Input: part model. Units: mm. Frame: model coordinates. Face numbers are marked on the shaded views. A direction names the side the tool comes from. Give positions to 0.01 mm unless a question says otherwise; leave off trailing zeros. Write each loop counter-clockwise with the first axis right and the second up, starting at its lowest first coordinate (ties: lowest second). Pieces come first, ordered by that corner, then holes.
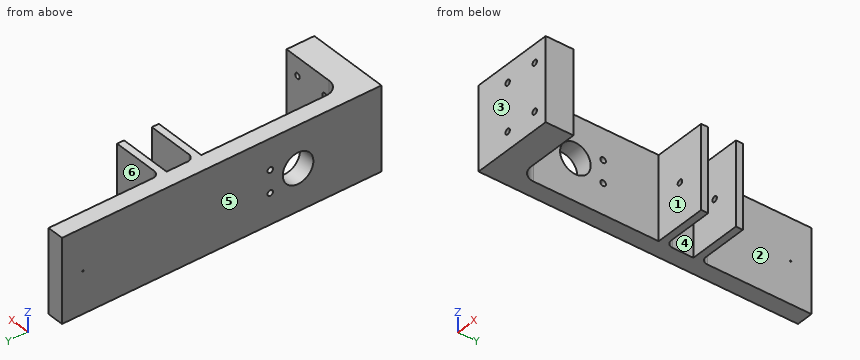
Autodesk Inventor part; units mm, degrees
ref_plane "YZ Plane" through (0, 0, 0) normal (1, 0, 0) x (0, 1, 0)
ref_plane "XZ Plane" through (0, 0, 0) normal (0, 1, 0) x (-1, 0, 0)
ref_plane "XY Plane" through (0, 0, 0) normal (0, 0, 1) x (1, 0, 0)
sketch "Эскиз1" plane through (0, 0, 0) normal (0, 1, 0) x (-1, 0, 0)
  line L0 (0, 0) -> (-60, 0)
  line L1 (-60, 0) -> (-60, -60)
  line L2 (-60, -60) -> (0, -60)
  line L3 (0, -60) -> (0, 0)
  dimension "d0" = 60
  dimension "d1" = 60
extrude "Выдавливание1" add sketch "Эскиз1" along normal blind 20
sketch "Эскиз2" plane through (0, 20, 0) normal (0, 1, 0) x (1, 0, 0)
  line L0 (0, 0) -> (60, 0)
  line L1 (0, 0) -> (12, 0)
  line L2 (12, 0) -> (12, 60)
  line L3 (60, 60) -> (0, 60)
  line L4 (0, 60) -> (0, 0)
  line L5 (0, 60) -> (0, 0)
  dimension "d4" = 12
extrude "Выдавливание2" add sketch "Эскиз2" along normal blind 260
sketch "Эскиз3" plane through (0, 20, 0) normal (0, 1, 0) x (1, 0, 0)
  point P0 (0, 0)
  point P1 (26, 13)
  point P2 (26, 47)
  point P3 (50.2241, 13)
  point P4 (50.2241, 47)
hole "Отверстие1" at (26, 20, -13) at (26, 20, -47) at (50.2241, 20, -13) at (50.2241, 20, -47) direction (0, -1, 0) diameter 4 depth 40 tip angle 118
sketch "Эскиз4" plane through (12, 20, 0) normal (1, 0, 0) x (0, 0, -1)
  point P0 (0, -20)
  point P1 (30, 88)
  dimension "d14" = 0
extrude "Выдавливание3" [suppressed]
sketch "Эскиз5" plane through (12, 20, 0) normal (1, 0, 0) x (0, 0, -1)
  point P0 (0, -20)
sketch "Эскиз6" plane through (0, 0, 0) normal (0, 0, 1) x (1, 0, 0)
  line L0 (0, 0) -> (0, 280)
  line L1 (12, 20) -> (12, 280)
sketch "Эскиз7" plane through (60, 0, -60) normal (0, 0, -1) x (-1, 0, 0)
  point P0 (60, 0)
sketch "Эскиз8" plane through (12, 20, 0) normal (1, 0, 0) x (0, 0, -1)
  circle A0 centre (30, 80) radius 11.5
  point P0 (0, -20)
  point P1 (0, 80)
  dimension "d17" = 23
extrude "Выдавливание4" cut sketch "Эскиз8" against normal blind 100
sketch "Эскиз9" plane through (0, 0, -60) normal (-1, 0, 0) x (0, 0, 1)
  circle A0 centre (29.731, 99.8395) radius 12.5286
  point P0 (60, 0)
  point P1 (0, 80)
extrude "Выдавливание5" add sketch "Эскиз9" against normal blind 12
sketch "Эскиз10" plane through (0, 0, -60) normal (-1, 0, 0) x (0, 0, 1)
  line L0 (0, 0) -> (0, 280)
  circle A0 centre (30, 60) radius 11
  circle A1 centre (22, 80) radius 2
  circle A2 centre (38, 80) radius 2
  point P0 (60, 0)
  point P1 (0, 60)
  point P2 (0, 80)
  point P3 (30, 80)
  dimension "d22" = 22
  dimension "d23" = 4
  dimension "d24" = 4
extrude "Выдавливание6" cut sketch "Эскиз10" against normal blind 12
sketch "Эскиз11" plane through (0, 0, 0) normal (0, -1, 0) x (1, 0, 0)
  point P0 (0, 0)
fillet "Сопряжение1" radius 10 1 edges at (12, 20, -30)
sketch "Эскиз12" plane through (0, 0, -60) normal (-1, 0, 0) x (0, 0, 1)
  line L0 (0, 120) -> (60, 120)
  line L1 (60, 120) -> (60, 125)
  line L2 (60, 125) -> (0, 125)
  line L3 (0, 125) -> (0, 120)
  point P0 (60, 0)
  dimension "d28" = 60
  dimension "d29" = 5
extrude "Выдавливание7" add sketch "Эскиз12" against normal blind 50
fillet "Сопряжение2" radius 5 1 edges at (12, 125, -30)
sketch "Эскиз13" plane through (50, 125, 0) normal (0, 1, 0) x (1, 0, 0)
  circle A0 centre (-19, 30) radius 2
  point P0 (-50, 0)
  dimension "d33" = 4
extrude "Выдавливание8" cut sketch "Эскиз13" against normal blind 50
sketch "Эскиз14" plane through (0, 0, -60) normal (-1, 0, 0) x (0, 0, 1)
  line L0 (0, 0) -> (0, 280)
  line L1 (0, 145) -> (60, 145)
  line L2 (60, 145) -> (60, 150)
  line L3 (60, 150) -> (0, 150)
  line L4 (0, 150) -> (0, 145)
  point P0 (60, 0)
  dimension "d36" = 60
  dimension "d37" = 5
extrude "Выдавливание9" add sketch "Эскиз14" against normal blind 50
fillet "Сопряжение3" radius 5 1 edges at (12, 150, -30)
sketch "Эскиз15" plane through (12, 145, -60) normal (0, -1, 0) x (1, 0, 0)
  circle A0 centre (19, 30) radius 2
  circle A1 centre (19, 30) radius 2
  circle A2 centre (19, 30) radius 2
  point P0 (-12, 60)
  point P1 (3.4297, 11.4015)
  dimension "d41" = 4
extrude "Выдавливание10" cut sketch "Эскиз15" against normal blind 50
sketch "Эскиз16" plane through (0, 0, -60) normal (-1, 0, 0) x (0, 0, 1)
  line L0 (0, 0) -> (0, 280)
  circle A0 centre (30, 215) radius 0.5
  point P0 (60, 0)
  point P1 (0, 215)
  point P2 (0, 215)
  dimension "d44" = 1
extrude "Выдавливание11" cut sketch "Эскиз16" against normal blind 100
sketch "Эскиз17" plane through (12, 280, 0) normal (1, 0, 0) x (0, 0, -1)
  point P0 (0, -280)
sketch "Эскиз18" plane through (12, 280, 0) normal (1, 0, 0) x (0, 0, -1)
  line L0 (0, -125) -> (0, 0)
  line L1 (60, -280) -> (60, 0)
  line L2 (0, -80) -> (0, -50)
  line L3 (0, -50) -> (5, -50)
  line L4 (5, -50) -> (5, -80)
  line L5 (5, -80) -> (0, -80)
  line L6 (0, -80) -> (0, -50)
  point P0 (0, -280)
  point P1 (30, -80)
  point P2 (30, -50)
  dimension "d47" = 5
extrude "Выдавливание12" add sketch "Эскиз18" along normal blind 44.5
sketch "Эскиз19" plane through (0, 0, 0) normal (0, 0, 1) x (1, 0, 0)
  circle A0 centre (52.5, 223) radius 2
  circle A1 centre (52.5, 207) radius 2
  point P0 (0, 0)
  point P1 (52.5, 215)
  dimension "d50" = 4
  dimension "d51" = 4
extrude "Выдавливание13" cut sketch "Эскиз19" against normal blind 45
fillet "Сопряжение4" radius 10 1 edges at (12, 215, -5)
sketch "Эскиз20" plane through (12, 280, 0) normal (1, 0, 0) x (0, 0, -1)
  line L0 (0, -280) -> (0, 0)
  line L1 (0, -50.033) -> (60, -50.033)
  line L2 (60, -280) -> (60, 0)
  line L3 (60, -50.033) -> (60, 0)
  line L4 (60, 0) -> (0, 0)
  line L5 (0, 0) -> (0, -50.033)
extrude "Выдавливание14" cut sketch "Эскиз20" against normal blind 100
sketch "Эскиз21" plane through (0, 0, 0) normal (0, 0, 1) x (1, 0, 0)
  line L0 (22, 230) -> (12, 230)
  line L1 (22, 200) -> (56.5, 200)
  line L2 (12, 230) -> (56.5, 230)
  line L3 (56.5, 230) -> (56.5, 200)
  line L4 (56.5, 200) -> (12, 200)
  line L5 (12, 200) -> (12, 230)
  point P0 (0, 0)
extrude "Выдавливание15" cut sketch "Эскиз21" against normal blind 100
properties part number "Подпора"
Q1. Section B-B, the plane y = 80. Return the cut outline in (x, z).
Q2. Section A-A, the plane x = 26. Return the cut outline in (y, z).
Q3. Mould query, pull axis Y, two halves, no side actions, for the marked faces 4, 5 and 6. Classes: +Y half, -Y half, draft (parallel to the pull), parting line (faces both ways), or undercut.
Q4. Pin query (flat end, axial travel): pin 1 (6.5 mm diameter, centred on x = 50.22, z = -47, fed in from +Y); pin 2 (16.5 mm diameter, centred on y = 138, z = -24, fed in from +X); pin 3 (6 mm diameter, centred on y = 168.5, z = -53, fed in from +X). Return the tip coordinate at first contact, or that it passes through.
Q5. Section C-C, the plane z = -13. Return the cut outline in (x, y), then the cut area to 3 significant figures.
Q6. Access query for the marked faces 1, 2 and 3. Directions: +Z, -Z, +X, -X, +Y, -Y. A direction counts if a zero-diameter tool reaches every point of the face in a straight line with its end or side. Return the directions, or none.
Q7. Material intervals for line 1 along Z through (x, y) = (26, 8); line 2 along Y through (x, z) = (2.5, -30); line 3 along Y through (x, z) = (49, -20.5), sorted ascending.
Q8. Section D-D, the plane x = 38.5. Return the cut outline in (y, z), then the cut area to 3 significant figures.
Solutions:
1. outline: (0, -60) - (12, -60) - (12, -40) - (0, -40) - close; (0, -36) - (12, -36) - (12, -24) - (0, -24) - close; (0, -20) - (12, -20) - (12, 0) - (0, 0) - close
2. outline: (0, -60) - (20, -60) - (20, -49) - (0, -49) - close; (0, -45) - (20, -45) - (20, -15) - (0, -15) - close; (0, -11) - (20, -11) - (20, 0) - (0, 0) - close; (120, -60) - (125, -60) - (125, 0) - (120, 0) - close; (145, -60) - (150, -60) - (150, 0) - (145, 0) - close
3. face 4: undercut
3. face 5: draft
3. face 6: +Y half
4. pin 1: stops at y = 150
4. pin 2: stops at x = 50
4. pin 3: stops at x = 12
5. outline: (0, 0) - (24, 0) - (24, 20) - (22, 20) arc R10 cw to (12, 30) - (12, 120) - (50, 120) - (50, 125) - (17, 125) arc R5 cw to (12, 130) - (12, 145) - (50, 145) - (50, 150) - (17, 150) arc R5 cw to (12, 155) - (12, 229.97) - (0, 229.97) - close; (28, 0) - (48.22, 0) - (48.22, 20) - (28, 20) - close; (52.22, 0) - (60, 0) - (60, 20) - (52.22, 20) - close
5. area: 3,970 mm2
6. face 1: +Z, -Z, +X
6. face 2: +Z, -Z, +X, +Y
6. face 3: +Z, -Z, +X, -X, -Y
7. line 1: z = -60 to -49, -45 to -15, -11 to 0
7. line 2: y = 0 to 49, 71 to 214.5, 215.5 to 229.97
7. line 3: y = 0 to 20, 120 to 125, 145 to 150
8. outline: (0, -60) - (20, -60) - (20, 0) - (0, 0) - close; (120, -60) - (125, -60) - (125, 0) - (120, 0) - close; (145, -60) - (150, -60) - (150, 0) - (145, 0) - close
8. area: 1,800 mm2
